Source: CAD feature listing. Evaluate the final solid. Frame: model axes, mm. A direction names the side the tool comes from. Round coordinates to 2 decimals unless told otherwise and drop trailing zeros. Loops run counter-clockwise (first coordinate to the right, second up) from the corner with the lowest first, then second, coordinate; pieces in that order, holes last. Notation, with made-up numbers: M 72,-14 L 85,-14 A25 cw 85,15 Z; hole C -33,33 d6. An arc over 180 degrees is marked long. Answer as a JSON object with one key per item and string values.
Autodesk Inventor part; units mm, degrees
ref_plane "YZ Plane" through (0, 0, 0) normal (1, 0, 0) x (0, 1, 0)
ref_plane "XZ Plane" through (0, 0, 0) normal (0, 1, 0) x (-1, 0, 0)
ref_plane "XY Plane" through (0, 0, 0) normal (0, 0, 1) x (1, 0, 0)
sketch "Sketch1" plane through (0, 0, 0) normal (0, 0, 1) x (1, 0, 0)
  line L0 (-1, 0) -> (13, 0)
  line L1 (0, -2.3) -> (0, 29.9)
  line L2 (6.5, 0) -> (6.5, 18)
  line L3 (6.5, 18) -> (8.5, 18)
  line L4 (8.5, 18) -> (8.5, 21)
  line L5 (8.5, 21) -> (6.5, 21)
  line L6 (6.5, 21) -> (6.5, 23)
  line L7 (6.5, 23) -> (10, 23)
  line L8 (10, 23) -> (10, 8)
  line L9 (10, 8) -> (8, 8)
  line L10 (8, 8) -> (8, 0)
  line L11 (8, 0) -> (6.5, 0)
  point P0 (0, 0)
  dimension "d0" = 13
  dimension "d1" = 16
  dimension "d2" = 20
  dimension "d3" = 8
  dimension "d4" = 23
  dimension "d5" = 2
  dimension "d6" = 3
  dimension "d7" = 2
revolve "Revolution1" add sketch "Sketch1" angle 360 about axis through (0, -10, 0) along (0, 1, 0)
sketch "Sketch2" plane through (0, 23, 0) normal (0, 1, 0) x (1, 0, 0)
  circle A0 centre (0, 0) radius 10
  circle A1 centre (0, 0) radius 6.5
  line L0 (-12, 0) -> (16, 0)
  line L1 (0, 12) -> (0, -16)
  line L2 (0, -14.4338) -> (-12.5, -7.2169)
  line L3 (-12.5, -7.2169) -> (-12.5, 7.2169)
  line L4 (-12.5, 7.2169) -> (0, 14.4338)
  line L5 (0, 14.4338) -> (12.5, 7.2169)
  line L6 (12.5, 7.2169) -> (12.5, -7.2169)
  line L7 (12.5, -7.2169) -> (0, -14.4338)
  dimension "d9" = 25
extrude "Extrusion1" add sketch "Sketch2" against normal blind 5 contours L0 L6 L7 L1 A0 | A0 L1 L2 L3 L4 L5 L6 L0
fillet "Fillet1" radius 3 6 edges at (0, 20.5, 14.4338) (-12.5, 20.5, 7.2169) (-12.5, 20.5, -7.2169) (0, 20.5, -14.4338) (12.5, 20.5, -7.2169) (12.5, 20.5, 7.2169)
chamfer "Chamfer1" distance 0.5 angle 45 1 edges at (-6.5, 0, 0)
chamfer "Chamfer2" distance 0.5 distance2 1 1 edges at (-8, 0, 0) measured on face at (7.5214, 0, 1.1966)
thread "Thread1"
properties part number "Packing Nut" material "Bronze, Soft Tin"
Item 1: Section C-C on y = 19.5. Return the cut outline in (x, z).
Answer sheet:
{"outline": "M -12.5,-5.48 A3 ccw -11,-8.08 L -1.5,-13.57 A3 ccw 1.5,-13.57 L 11,-8.08 A3 ccw 12.5,-5.48 L 12.5,5.48 A3 ccw 11,8.08 L 1.5,13.57 A3 ccw -1.5,13.57 L -11,8.08 A3 ccw -12.5,5.48 Z; hole C 0,0 d17"}
Item 2: Access query for faces 5 (the cylindrical face through (-2.17, 12.93, -9.76)), 6 (the flat face through (6.317, 20.535, 10.787)), 7 (the cylindrical face through (4.57, 19.521, -7.167)). Directions: +Z, -Z, +X, -X, +Y, -Y. A direction counts if a zero-diameter tool reaches every point of the face in a straight line with its end or side. Return the directions, or none.
Answer sheet:
{"face 5": "-Y", "face 6": "+Z, +X, +Y, -Y", "face 7": "none"}
Item 3: Contact query for flat-ended pins moving along their axis: pin 1 Ø6 at (x, y) = (0.5, 14.5) entering from -Z; pin 2 Ø4 at (y, z) = (5, -3.5) entering from +X; pin 3 Ø2 at (y, z) = (20, 11) entering from +X; pin 4 Ø10 at (x, z) = (-0.5, 0) entering from -Y. Output: stop coordinate, or through.
Answer sheet:
{"pin 1": "stops at z = -10", "pin 2": "stops at x = 7.86", "pin 3": "stops at x = 7.68", "pin 4": "passes through"}
Item 4: Line query: probe 1 along Z at (x, y) = (0, 22.4); probe 2 along Z at (x, y) = (0, 12); probe 3 along Y at (x, z) = (-2.5, -11). Output: solid intervals per line, ascending. Write a range as from..to.
Answer sheet:
{"probe 1": "z = -13.97..-6.5, 6.5..13.97", "probe 2": "z = -10..-6.5, 6.5..10", "probe 3": "y = 18..23"}
Item 5: Section B-B on z = 0. Return the cut outline in (x, y).
Answer sheet:
{"outline": "M -12.5,18 L -10,18 L -10,8 L -8,8 L -8,1 L -7.5,0 L -7,0 L -6.5,0.5 L -6.5,18 L -8.5,18 L -8.5,21 L -6.5,21 L -6.5,23 L -12.5,23 Z; M 6.5,0.5 L 7,0 L 7.5,0 L 8,1 L 8,8 L 10,8 L 10,18 L 12.5,18 L 12.5,23 L 6.5,23 L 6.5,21 L 8.5,21 L 8.5,18 L 6.5,18 Z"}
Item 6: Pull-direction query (Y, two-part tool) for faces 1 (the flat face through (-0.1, 18, -10.4)), 2 (the flat face through (4.4, 21, 5)), 3 (the flat face through (-6.317, 20.535, -10.787)), 4 (the flat face through (-6, 23, -3)); classes: pulls with the +Y half, pulls with the -Y half, needs draft (parallel to the pull), parting line crosses it, or undercut.
Answer sheet:
{"face 1": "pulls with the -Y half", "face 2": "undercut", "face 3": "needs draft", "face 4": "pulls with the +Y half"}
Item 7: Section D-D on x = -9.5. Return the cut outline in (y, z).
Answer sheet:
{"outline": "M 8,-3.12 L 18,-3.12 L 18,-8.95 L 23,-8.95 L 23,8.95 L 18,8.95 L 18,3.12 L 8,3.12 Z"}
Item 8: Section A-A on x = 0. Return the cut outline in (y, z).
Answer sheet:
{"outline": "M 0,-7.5 L 1,-8 L 8,-8 L 8,-10 L 18,-10 L 18,-13.97 L 23,-13.97 L 23,-6.5 L 21,-6.5 L 21,-8.5 L 18,-8.5 L 18,-6.5 L 0.5,-6.5 L 0,-7 Z; M 0,7 L 0.5,6.5 L 18,6.5 L 18,8.5 L 21,8.5 L 21,6.5 L 23,6.5 L 23,13.97 L 18,13.97 L 18,10 L 8,10 L 8,8 L 1,8 L 0,7.5 Z"}
